Read the model definition and answer for the solid it produces. Units are mm, in the model's axes. Coordinates: 2 decimals unless noted, no trailing zeros. Loops run counter-clockwise (first coordinate to the right, second up) from the corner with the lowest first, then second, coordinate; pieces in that order, holes last.
Solid Edge part; units mm, degrees
sketch "Sketch1" plane through (0, 0, 0) normal (0, 0, 1) x (1, 0, 0)
  line L0 (-175, -100) -> (175, -100)
  line L1 (175, -100) -> (175, 100)
  line L2 (175, 100) -> (-175, 100)
  line L3 (-175, 100) -> (-175, -100)
  dimension "D1" = 175
  dimension "D2" = 175
extrude "Protrusion1" add sketch "Sketch1" along normal blind 3
sketch "Sketch2" plane through (0, 0, 3) normal (0, 0, 1) x (1, 0, 0)
  line L0 (-69, 100) -> (-91, 100)
  line L1 (-91, 100) -> (-91, 72)
  line L2 (-91, 72) -> (-69, 72)
  line L3 (-69, 72) -> (-69, 100)
  line L4 (-11, 72) -> (11, 72)
  line L5 (11, 72) -> (11, 100)
  line L6 (11, 100) -> (-11, 100)
  line L7 (-11, 100) -> (-11, 72)
  line L8 (-175, -11) -> (-103, -11)
  line L9 (-103, -11) -> (-103, 11)
  line L10 (-103, 11) -> (-175, 11)
  line L11 (-175, 11) -> (-175, -11)
  dimension "D1" = 11
  dimension "D2" = 11
  dimension "D3" = 69
extrude "Cutout1" cut sketch "Sketch2" against normal up to next
sketch "Sketch3" plane through (0, 0, 3) normal (0, 0, 1) x (1, 0, 0)
  line L0 (-150, 100) -> (-120, 100)
  line L1 (-120, 100) -> (-125, 112)
  line L2 (-125, 112) -> (-145, 112)
  line L3 (-145, 112) -> (-150, 100)
  dimension "D1" = 145
  dimension "D2" = 150
  dimension "D3" = 125
extrude "Protrusion2" add sketch "Sketch3" against normal up to vertex (3 mm away)
hole "Hole_1" at (-135, 106, 3) direction (0, 0, -1) diameter 4.3 end up to next
mirror "Mirror1" about plane through (0, 0, 0) normal (0, -1, 0) of "Cutout1", "Protrusion2", "Hole_1"
mirror "Mirror2" about plane through (0, 0, 0) normal (1, 0, 0) of "Cutout1", "Protrusion2", "Hole_1", "Mirror1"
properties material "Glass, general industrial"
Q1. A cutting plane is placed at D-D (y = -5.5). Give the vertices of the cut face in (x, z).
Findings below:
outline: (-103, 0) - (103, 0) - (103, 3) - (-103, 3) - close
Q2. A cutting plane is placed at C-C (x = -83). Give the vertices of the cut face in (y, z).
Findings below:
outline: (-72, 0) - (72, 0) - (72, 3) - (-72, 3) - close
Q3. Flat-ended cylindrical pins translate along their axes: pin 1 Ø1.5 at (x, z) = (-83, 1.5) entering from -Y; pin 2 Ø1.5 at (x, z) = (98.5, 1) entering from +Y. Find the tip coordinate at first contact, or state that the pin passes through.
Findings below:
pin 1: stops at y = -72
pin 2: stops at y = 100
Q4. Straight lines are drawn through the part: probe 1 along Y at (x, z) = (135, 0.9); probe 2 along Y at (x, z) = (151, 2.05); probe 3 along X at (y, z) = (106, 2.05). For each, find the intervals that lie inside material, in ascending order.
Findings below:
probe 1: y = -112 to -108.15, -103.85 to -11, 11 to 103.85, 108.15 to 112
probe 2: y = -100 to -11, 11 to 100
probe 3: x = -147.5 to -137.15, -132.85 to -122.5, 122.5 to 132.85, 137.15 to 147.5
Q5. A cutting plane is placed at B-B (z = 1). Count the separate pieces of the cut face and the enclosed holes in it, then the cut area to 3 significant figures.
Findings below:
separate pieces: 1
enclosed holes: 4
area: 64,300 mm2
Q6. A cutting plane is placed at A-A (y = -80). Give the vertices of the cut face in (x, z), then the cut area to 3 significant figures.
Findings below:
outline: (-175, 0) - (-91, 0) - (-91, 3) - (-175, 3) - close; (-69, 0) - (-11, 0) - (-11, 3) - (-69, 3) - close; (11, 0) - (69, 0) - (69, 3) - (11, 3) - close; (91, 0) - (175, 0) - (175, 3) - (91, 3) - close
area: 852 mm2
